Can you work these out from the model? Positions are in its coordinate system, mm. A direction names the side the tool comes from. Coordinates: 2 decimals unless noted, no trailing zeros. Order: outer loops, then holes, each group sorted by start corner. A loop starts at its lowest first (then second) coordinate and runs counter-clockwise, first axis right, second up. Notation, with made-up numbers: (-5.5, 79.5) -> (10.5, 79.5) arc R26 cw to (10.5, 99.5) -> close; hole circle Ø1 at (13, 72). An arc over 180 degrees is marked (long way). Answer in a Markdown table with one row per item. Add a question column.
1. If I drill on line 1 along Y through (x, z) = (0, 4.25); line 2 along X through (y, z) = (3, 6); line 3 along Z through (x, y) = (-19.5, 12.5), over which ranges is the centre line in solid material (lowest first)? Write a range as [from, to].
2. We'd pull the mould along X, two halves only. Please class faces 1 (the face through (-3, 24, 8)), 2 (the face through (-3, -20, 18)), 3 (the face through (20, 14.514, 13.07)), 4 (the face through (-17, 18, 13)): pulls with the +X half, pulls with the -X half, needs draft (parallel to the pull), parting line crosses it, or undercut.
3. Imagine slicing it at A-A on x = 0. Write out the boundary of the cut face in (y, z), plus the area to 3 significant figures.
4. Will these pins go through, and if not, where does the flat tip stop? pin 1 (10 mm diameter, centred on x = 8.5, y = -5.5, fed in from +Z); pin 2 (5 mm diameter, centred on x = -3, y = -24.5, fed in from +Z); pin 3 (3 mm diameter, centred on y = 3.5, z = 2, fed in from -X); pin 4 (2 mm diameter, centred on x = 17.5, z = 13, fed in from +Y).
5. Imagine slicing it at D-D on x = -16.5. Write out the boundary of the cut face in (y, z) (3 decimals), plus the area to 3 significant figures.
6. On a 3-axis mill with a long thin cutter (end or side, diameter ignored), from which of +Z, -Z, +X, -X, +Y, -Y can I reach the whole of each face in a straight line? I mean faces 5 (the face through (-16.86, -17.23, 11.82)), 6 (the face through (-21.6, 10.71, 11.82)), 7 (the face through (20.074, 13.349, 11.819)), 8 (the face through (-6.492, -23.216, 11.819)), 9 (the face through (17, -18, 8)). Say none if no direction works.
7. Imagine slicing it at B-B on y = 9. Write out the boundary of the cut face in (x, z), plus the area to 3 significant figures.
8. Imagine slicing it at C-C on x = 16. Write out the boundary of the cut face in (y, z).
from build123d import *

# Parameters (mm, degrees)
SKETCH1_R           = 27.5
SKETCH1_R_2         = 20
BOSS_EXTRUDE1_DEPTH = 8
SKETCH2_R           = 22
SKETCH2_R_2         = 20
BOSS_EXTRUDE2_DEPTH = 10
BOSS_EXTRUDE3_DEPTH = 1
CIRPATTERN1_COUNT   = 15


with BuildPart() as part:
    # Sketch1 → Boss-Extrude1 (new body)
    with BuildSketch(Plane.XY):
        Circle(SKETCH1_R)
        Circle(SKETCH1_R_2, mode=Mode.SUBTRACT)
    extrude(amount=BOSS_EXTRUDE1_DEPTH)

    # Sketch2 → Boss-Extrude2 (add)
    with BuildSketch(Plane.XY.offset(8)):
        Circle(SKETCH2_R)
        Circle(SKETCH2_R_2, mode=Mode.SUBTRACT)
    extrude(amount=BOSS_EXTRUDE2_DEPTH)

    # Sketch3 → Boss-Extrude3 (add, symmetric)
    with BuildSketch(Plane(origin=(0, 0, 0), x_dir=(1, 0, 0), z_dir=(0, 1, 0))):
        Polygon((-22, -18), (-27.5, -8), (-22, -8), (-20.5, -8), (-20.5, -18), align=None)
    boss_extrude3 = extrude(amount=BOSS_EXTRUDE3_DEPTH, both=True)

    # CirPattern1: Boss-Extrude3 ×15 about axis
    cirpattern1_axis = Axis((0, 0, 0), (0, 0, 1))
    for i in range(1, CIRPATTERN1_COUNT):
        add(boss_extrude3.rotate(cirpattern1_axis, i * 360 / CIRPATTERN1_COUNT))


solid = part.part
Answers follow:
| question | item | result |
|---|---|---|
| 1 | line 1 | y = [-27.5, -20], [20, 27.5] |
| 1 | line 2 | x = [-27.34, -19.77], [19.77, 27.34] |
| 1 | line 3 | z = [0, 8] |
| 2 | face 1 | undercut |
| 2 | face 2 | needs draft |
| 2 | face 3 | pulls with the +X half |
| 2 | face 4 | pulls with the -X half |
| 3 | outline | (-27.5, 0) -> (-20, 0) -> (-20, 18) -> (-22, 18) -> (-22, 8) -> (-27.5, 8) -> close; (20, 0) -> (27.5, 0) -> (27.5, 8) -> (22, 8) -> (22, 18) -> (20, 18) -> close |
| 3 | area | 160 mm² |
| 4 | pin 1 | passes through |
| 4 | pin 2 | stops at z = 8 |
| 4 | pin 3 | stops at x = -27.43 |
| 4 | pin 4 | stops at y = 14.68 |
| 5 | outline | (-22, 0) -> (-11.303, 0) -> (-11.303, 18) -> (-14.552, 18) -> (-14.552, 8) -> (-16.831, 8) -> (-16.831, 15.185) -> (-19.82, 11.146) -> (-19.82, 8) -> (-22, 8) -> close; (11.303, 0) -> (22, 0) -> (22, 8) -> (19.82, 8) -> (19.82, 11.146) -> (16.831, 15.185) -> (16.831, 8) -> (14.552, 8) -> (14.552, 18) -> (11.303, 18) -> close |
| 5 | area | 267 mm² |
| 6 | face 5 | +Z, -X |
| 6 | face 6 | +Z, +Y |
| 6 | face 7 | +Z, +X |
| 6 | face 8 | +Z, -Y |
| 6 | face 9 | +Z |
| 7 | outline | (-25.99, 0) -> (-17.86, 0) -> (-17.86, 18) -> (-20.07, 18) -> (-22.67, 13.68) -> (-22.67, 8) -> (-25.99, 8) -> close; (17.86, 0) -> (25.99, 0) -> (25.99, 8) -> (20.07, 8) -> (20.07, 18) -> (17.86, 18) -> close |
| 7 | area | 195 mm² |
| 8 | outline | (-22.37, 0) -> (-12, 0) -> (-12, 18) -> (-15.1, 18) -> (-15.1, 8) -> (-22.37, 8) -> close; (12, 0) -> (22.37, 0) -> (22.37, 8) -> (15.1, 8) -> (15.1, 18) -> (12, 18) -> close |
